Can you work these out from the model? Positions are in its coordinate system, mm. A direction names the side the tool comes from. Give positions to 0.01 mm unless a question says otherwise; leave off trailing zeros. Write each loop counter-clockwise with the first axis right and the second up, starting at its lowest first coordinate (ties: lowest second). Pieces come first, ordered by that corner, then holes.
```python
from build123d import *

# Parameters (mm, degrees)
EXTRUDE1_DEPTH = 16
EXTRUDE6_DEPTH = 12
CHAMFER1_SIZE  = 2
SKETCH3_R      = 1.5
EXTRUDE7_DEPTH = 4


with BuildPart() as part:
    # Sketch1 → Extrude1 (new body)
    with BuildSketch(Plane.XY):
        Polygon((16.5, -10.5), (25, -10.5), (25, -14.5), (-25, -14.5), (-25, -10.5), (-16.5, -10.5), (-16.5, 14.5), (16.5, 14.5), align=None)
    extrude(amount=-EXTRUDE1_DEPTH)

    # Sketch2 → Extrude6 (cut)
    with BuildSketch(Plane.XY):
        Polygon((1, 14.5), (-1, 14.5), (-1, 4.5), (-16.5, 4.5), (-16.5, 2.5), (16.5, 2.5), (16.5, 4.5), (1, 4.5), align=None)
    extrude(amount=-EXTRUDE6_DEPTH, mode=Mode.SUBTRACT)

    # Chamfer1
    chamfer1_edges = [part.edges().sort_by_distance(p)[0] for p in [
        (-1, 9.5, 0),
        (8.75, 4.5, 0),
        (-8.75, 4.5, 0),
        (0, 2.5, 0),
        (1, 9.5, 0),
    ]]
    chamfer(chamfer1_edges, length=CHAMFER1_SIZE)

    # Sketch3 → Extrude7 (cut)
    with BuildSketch(Plane.XZ.offset(14.5)):
        with Locations((-20.5, -8)):
            Circle(SKETCH3_R)
        with Locations((20.5, -8)):
            Circle(SKETCH3_R)
    extrude(amount=-EXTRUDE7_DEPTH, mode=Mode.SUBTRACT)


solid = part.part
```
1) Suppose I cut it at D-D on x = 6.5. Write out the boundary of the cut face in (y, z), plus the area to 3 significant figures.
Values follow:
outline: (-14.5, -16) - (14.5, -16) - (14.5, 0) - (6.5, 0) - (4.5, -2) - (4.5, -12) - (2.5, -12) - (2.5, -2) - (0.5, 0) - (-14.5, 0) - close
area: 436 mm2
2) Suppose I cut it at A-A on z = -8. Write out the boundary of the cut face in (x, y), plus the area to 3 significant figures.
Values follow:
outline: (-25, -14.5) - (-22, -14.5) - (-22, -10.5) - (-25, -10.5) - close; (-19, -14.5) - (19, -14.5) - (19, -10.5) - (16.5, -10.5) - (16.5, 2.5) - (-16.5, 2.5) - (-16.5, -10.5) - (-19, -10.5) - close; (-16.5, 4.5) - (-1, 4.5) - (-1, 14.5) - (-16.5, 14.5) - close; (1, 4.5) - (16.5, 4.5) - (16.5, 14.5) - (1, 14.5) - close; (22, -14.5) - (25, -14.5) - (25, -10.5) - (22, -10.5) - close
area: 915 mm2
3) Suppose I cut it at C-C on y = -12. Write out the boundary of the cut face in (x, z).
Values follow:
outline: (-25, -16) - (25, -16) - (25, 0) - (-25, 0) - close; hole circle Ø3 at (-20.5, -8); hole circle Ø3 at (20.5, -8)
4) If we mould it in two halves opening along Z, with no side actions, what happens to faces 1 (the face through (0, 2.5, -7)), 2 (the face through (8.9, 5.5, -1)), 3 (the face through (19.3, -12.5, -8.9))? For each: +Z half, -Z half, draft (parallel to the pull), parting line (faces both ways), or undercut.
Values follow:
face 1: draft
face 2: +Z half
face 3: undercut
5) Please list where these lines run through material, in increasing order: L1, parallel to Y at x = -6.5, z = -8.5; L2, parallel to X at y = 8.5, z = -9.75; L3, parallel to Z at x = -20.5, y = -12.8.
Values follow:
L1: y = -14.5 to 2.5, 4.5 to 14.5
L2: x = -16.5 to -1, 1 to 16.5
L3: z = -16 to -9.5, -6.5 to 0
6) For pin 1 Ø1.5 at (y, z) = (9, -7) entering from +X; pin 2 Ø3 at (x, z) = (0.5, -9.5) entering from +Y; pin 3 Ø5 at (y, z) = (9.5, -8) entering from -X, each with a flat end and sliding along its axis, tell me the tip position at first contact or that it passes through.
Values follow:
pin 1: stops at x = 16.5
pin 2: stops at y = 14.5
pin 3: stops at x = -16.5
7) Suppose I cut it at B-B on x = 20.5. Write out the boundary of the cut face in (y, z).
Values follow:
outline: (-14.5, -16) - (-10.5, -16) - (-10.5, -9.5) - (-14.5, -9.5) - close; (-14.5, -6.5) - (-10.5, -6.5) - (-10.5, 0) - (-14.5, 0) - close
8) For faces 4 (the face through (-16.5, 2, -8)), 5 (the face through (16.5, 2, -8)), 6 (the face through (0, -14.5, -8)), 7 (the face through (-1, 10, -7)), 8 (the face through (-9, 4.5, -7)), which set-ups out of +Z, -Z, +X, -X, +Y, -Y let a thin tool reach every point of the face, with its end or its side?
Values follow:
face 4: +Z, -Z, -X, +Y
face 5: +Z, -Z, +X, +Y
face 6: +Z, -Z, +X, -X, -Y
face 7: +Z, +Y
face 8: +Z, +X, -X
